Check sheet for the modelled part. Datum: model origin and axes. Units: mm. A direction names the side the tool comes from. Round coordinates to 2 decimals unless told otherwise and drop trailing zeros. Loops run counter-clockwise (first coordinate to the right, second up) from the corner with the lowest first, then second, coordinate; pieces in that order, holes last. Notation, with made-up numbers: (70, -17.5) -> (94, -17.5) arc R5 cw to (94, -8.5) -> close; hole circle Ø9 at (-14.5, 34.25). An arc over 180 degrees is marked (long way). One line per item, written item: value. Start each with the question number.
1. Cross-section at C-C on x = 0. Record the cut outline in (y, z).
2. Cross-section at A-A on y = 1.35. Record the cut outline in (x, z), then the cut area to 3 significant figures.
3. Go/stop test with flat-tipped pins: pin 1 (0.6 mm diameter, centred on x = 11, y = 2, fed in from +Z); pin 2 (1.5 mm diameter, centred on y = 3.5, z = -17.5, fed in from -X); pin 3 (1 mm diameter, centred on x = -1, y = 2.5, fed in from -Z) (3 decimals). Record where each tip stops, or that it passes through.
4. Set-up check for faces 1 (the face through (10, 2, -6)), 2 (the face through (11, 3, -30)): record each of +Z, -Z, +X, -X, +Y, -Y from which the full face is reachable in a straight line by a thin tool's end or side.
5. Material ranges on L1, parallel to X at y = 1.75, z = -12; L2, parallel to Z at x = 2.25, y = 2.1; L3, parallel to Z at x = 8.25, y = 4.65, recorded low to high.
6. Cross-section at B-B on z = -10. Record the cut outline in (x, y).
from build123d import *

# Parameters (mm, degrees)
BOSS_EXTRUDE4_DEPTH = 5
BOSS_EXTRUDE5_DEPTH = 5


with BuildPart() as part:
    # Sketch4 → Boss-Extrude4 (new body)
    with BuildSketch(Plane(origin=(0, 0, 0), x_dir=(1, 0, 0), z_dir=(0, 1, 0))):
        Polygon((-10, 15), (10, 30), (10, 15), (10, -15), (-10, -15), align=None)
    extrude(amount=BOSS_EXTRUDE4_DEPTH)

    # Sketch6 → Boss-Extrude5 (add)
    with BuildSketch(Plane(origin=(0, 5, 0), x_dir=(1, 0, 0), z_dir=(0, 1, 0))):
        with BuildLine():
            Line((10, 30), (11.25, 30))
            ThreePointArc((11.25, 30), (11.426776695, 29.926776695), (11.5, 29.75))
            Line((11.5, 29.75), (11.5, 28))
            ThreePointArc((11.5, 28), (11.353553391, 27.646446609), (11, 27.5))
            Line((11, 27.5), (10.5, 27.5))
            ThreePointArc((10.5, 27.5), (10.146446609, 27.353553391), (10, 27))
            Line((10, 27), (10, 30))
        make_face()
    extrude(amount=-BOSS_EXTRUDE5_DEPTH)


solid = part.part
Taken from the geometry:
1. outline: (0, -22.5) -> (5, -22.5) -> (5, 15) -> (0, 15) -> close
2. outline: (-10, -15) -> (10, -30) -> (11.25, -30) arc R0.25 ccw to (11.5, -29.75) -> (11.5, -28) arc R0.5 ccw to (11, -27.5) -> (10.5, -27.5) arc R0.5 cw to (10, -27) -> (10, 15) -> (-10, 15) -> close
2. area: 754 mm2
3. pin 1: stops at z = -27.5
3. pin 2: stops at x = -7.67
3. pin 3: stops at z = -22.125
4. face 1: +Z, +X, +Y, -Y
4. face 2: -Z, +X, -X, +Y, -Y
5. L1: x = -10 to 10
5. L2: z = -24.19 to 15
5. L3: z = -28.69 to 15
6. outline: (-10, 0) -> (10, 0) -> (10, 5) -> (-10, 5) -> close
